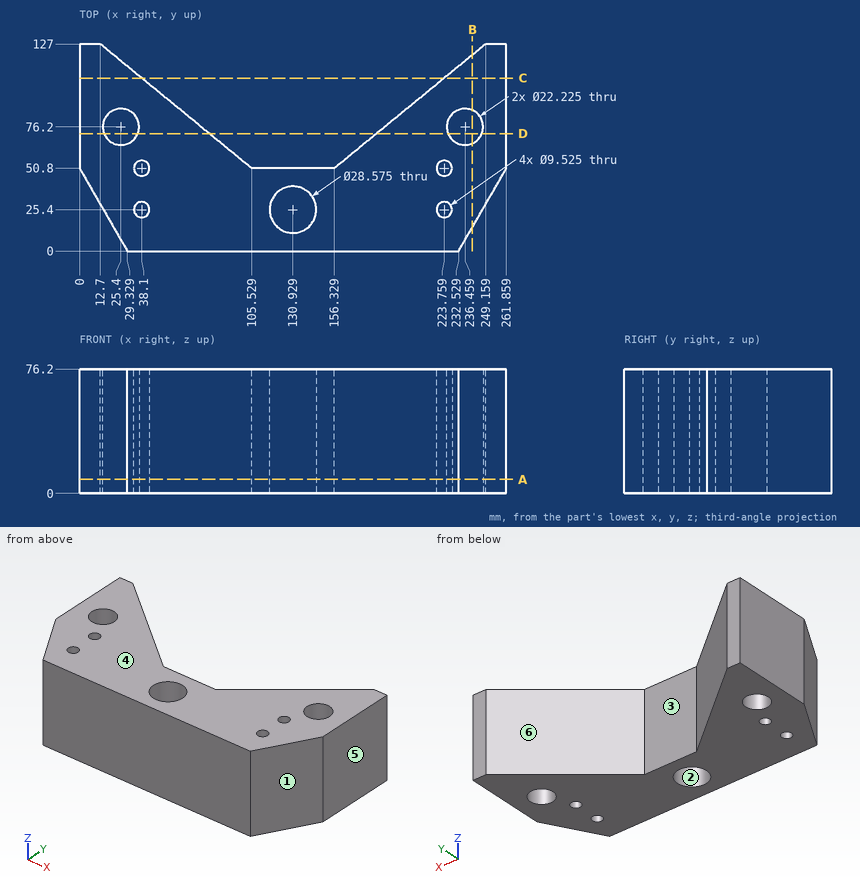
Verification items for this drawing (mm, ordinates from the low corner). A direction names the side the tool comes from. Coordinates: 2 decimals unless noted, no trailing zeros. Order: outer loops, then holes, each group sorted by start corner. A loop starts at its lowest first (then second) coordinate and runs counter-clockwise, first axis right, second up. Notation, with made-up numbers: M 30.25,56.5 L 45.25,56.5 A21 cw 45.25,63.5 Z; hole C -30.5,-3 d2. An arc over 180 degrees is marked long. Answer as a JSON object with one key per item and string values.
Q1. Release check for a two-part mould opening along X. For the marked faces 1, 2, 3 and 4 record: released by +X, released by -X, zero draft, split by the parting line, or undercut.
Results are:
{"face 1": "released by +X", "face 2": "undercut", "face 3": "undercut", "face 4": "zero draft"}
Q2. Tool access check on the marked faces 5 and 6. Record the directions out of +Z, -Z, +X, -X, +Y, -Y that give a thin tool (end or side, any length) a straight path to the whole face; none if there is none.
Results are:
{"face 5": "+Z, -Z, +X, +Y, -Y", "face 6": "+Z, -Z, +Y"}
Q3. Cross-section at A-A on z = 8.5. Record the cut outline in (x, y) (1 decimal), and give its area (3 significant figures).
Results are:
{"outline": "M 0,50.8 L 29.3,0 L 232.5,0 L 261.9,50.8 L 261.9,127 L 249.2,127 L 156.3,50.8 L 105.5,50.8 L 12.7,127 L 0,127 Z; hole C 25.4,76.2 d22.2; hole C 38.1,25.4 d9.5; hole C 38.1,50.8 d9.5; hole C 130.9,25.4 d28.6; hole C 223.8,25.4 d9.5; hole C 223.8,50.8 d9.5; hole C 236.5,76.2 d22.2", "area": "19,100 mm²"}
Q4. Cross-section at D-D on y = 72. Record the cut outline in (x, z), and give its area (3 significant figures).
Results are:
{"outline": "M 0,0 L 15.11,0 L 15.11,76.2 L 0,76.2 Z; M 35.69,0 L 79.7,0 L 79.7,76.2 L 35.69,76.2 Z; M 182.16,0 L 226.17,0 L 226.17,76.2 L 182.16,76.2 Z; M 246.75,0 L 261.86,0 L 261.86,76.2 L 246.75,76.2 Z", "area": "9,010 mm²"}
Q5. Depth check by flat-ended pin: pin 1 Ø15 at (x, z) = (128, 31.5) entering from +Y; pin 2 Ø1 at (x, z) = (171, 27.5) entering from +Y. Enter the tip coordinate at first touch or a pass-through.
Results are:
{"pin 1": "stops at y = 50.8", "pin 2": "stops at y = 63.25"}
Q6. Scan lines: line 1 (X direction, y = 25.4, z = 33.5) (1 decimal); line 2 (X direction, y = 68, z = 68.5) (1 decimal); line 3 (Y direction, x = 38.1, z = 46). Record each from-to range of solid material in increasing order.
Results are:
{"line 1": "x = 14.7 to 33.3, 42.9 to 116.6, 145.2 to 219, 228.5 to 247.2", "line 2": "x = 0 to 17.9, 32.9 to 84.6, 177.3 to 229, 244 to 261.9", "line 3": "y = 0 to 20.64, 30.16 to 46.04, 55.56 to 106.15"}
Q7. Cross-section at C-C on y = 106. Record the cut outline in (x, z).
Results are:
{"outline": "M 0,0 L 38.28,0 L 38.28,76.2 L 0,76.2 Z; M 223.58,0 L 261.86,0 L 261.86,76.2 L 223.58,76.2 Z"}
Q8. Cross-section at B-B on x = 241. Record the cut outline in (y, z).
Results are:
{"outline": "M 14.67,0 L 66.06,0 L 66.06,76.2 L 14.67,76.2 Z; M 86.34,0 L 120.3,0 L 120.3,76.2 L 86.34,76.2 Z"}
